```python
from build123d import *

# Parameters (mm, degrees)
SKETCH2_W           = 74.46
SKETCH2_H           = 52.500000064
SKETCH2_R           = 1
BOSS_EXTRUDE1_DEPTH = 2


with BuildPart() as part:
    # Sketch2 → Boss-Extrude1 (new body)
    with BuildSketch(Plane.XY):
        with Locations((51.585490461, 10.250000032)):
            Rectangle(SKETCH2_W, SKETCH2_H)
        with Locations((66.855490461, 35.000000064)):
            Circle(SKETCH2_R, mode=Mode.SUBTRACT)
        with Locations((15.855490461, 5.000000064)):
            Circle(SKETCH2_R, mode=Mode.SUBTRACT)
        with Locations((85.815490461, 35.000000064)):
            Circle(SKETCH2_R, mode=Mode.SUBTRACT)
        with Locations((85.815490461, -5.000000191)):
            Circle(SKETCH2_R, mode=Mode.SUBTRACT)
        with BuildLine():
            ThreePointArc((71.255490461, -4.000000191), (70.255490461, -5.000000191), (71.255490461, -6.000000191))
            ThreePointArc((71.255490461, -6.000000191), (72.255490461, -5.000000191), (71.255490461, -4.000000191))
        make_face(mode=Mode.SUBTRACT)
        with BuildLine():
            ThreePointArc((18.355490461, -13.5), (19.355490461, -14.5), (20.355490461, -13.5))
            ThreePointArc((20.355490461, -13.5), (19.355490461, -12.5), (18.355490461, -13.5))
        make_face(mode=Mode.SUBTRACT)
        with BuildLine():
            ThreePointArc((18.355490461, -8.5), (19.355490461, -9.5), (20.355490461, -8.5))
            ThreePointArc((20.355490461, -8.5), (19.355490461, -7.5), (18.355490461, -8.5))
        make_face(mode=Mode.SUBTRACT)
        with BuildLine():
            ThreePointArc((17.855490461, 0.500000064), (16.855490461, -0.499999936), (17.855490461, -1.499999936))
            ThreePointArc((17.855490461, -1.499999936), (18.855490461, -0.499999936), (17.855490461, 0.500000064))
        make_face(mode=Mode.SUBTRACT)
        with BuildLine():
            ThreePointArc((24.855490461, 0.500000064), (23.855490461, -0.499999936), (24.855490461, -1.499999936))
            ThreePointArc((24.855490461, -1.499999936), (25.855490461, -0.499999936), (24.855490461, 0.500000064))
        make_face(mode=Mode.SUBTRACT)
        with BuildLine():
            ThreePointArc((60.855490461, -13.5), (61.855490461, -14.5), (62.855490461, -13.5))
            ThreePointArc((62.855490461, -13.5), (61.855490461, -12.5), (60.855490461, -13.5))
        make_face(mode=Mode.SUBTRACT)
        with BuildLine():
            ThreePointArc((62.855490461, -8.5), (61.855490461, -7.5), (60.855490461, -8.5))
            ThreePointArc((60.855490461, -8.5), (61.855490461, -9.5), (62.855490461, -8.5))
        make_face(mode=Mode.SUBTRACT)
        with BuildLine():
            ThreePointArc((71.255490461, 34.000000064), (72.255490461, 35.000000064), (71.255490461, 36.000000064))
            ThreePointArc((71.255490461, 36.000000064), (70.255490461, 35.000000064), (71.255490461, 34.000000064))
        make_face(mode=Mode.SUBTRACT)
    extrude(amount=BOSS_EXTRUDE1_DEPTH)


solid = part.part
```
Check sheet for the modelled part. Datum: model origin and axes. Units: mm. Give positions to 0.01 mm unless a question says otherwise; leave off trailing zeros. Loops run counter-clockwise (first coordinate to the right, second up) from the corner with the lowest first, then second, coordinate; pieces in that order, holes last. Notation, with made-up numbers: M 19.25,1 L 34.25,1 A25 ccw 34.25,23 Z; hole C 3.5,74.5 d2. An arc over 180 degrees is marked long. Answer in a Markdown table with one row per item.
1) Mould release check, pull along Y, two halves, no side actions. Record for faces 1 (the face through (51, 36.5, 1)), 2 (the face through (88.815, 10, 1)), 3 (the face through (72.247, -4.87, 0.986)), 4 (the face through (18.62, -7.82, 0.99)): released by +Y, released by -Y, zero draft, split by the parting line, or undercut.
Solutions:
| item | result |
|---|---|
| face 1 | released by +Y |
| face 2 | zero draft |
| face 3 | undercut |
| face 4 | undercut |
2) Cross-section at A-A (y = 35). Enter the section's corners in (x, z).
Solutions:
| item | result |
|---|---|
| outline | M 14.36,0 L 65.86,0 L 65.86,2 L 14.36,2 Z; M 67.86,0 L 70.26,0 L 70.26,2 L 67.86,2 Z; M 72.26,0 L 84.82,0 L 84.82,2 L 72.26,2 Z; M 86.82,0 L 88.82,0 L 88.82,2 L 86.82,2 Z |
3) Cross-section at B-B (y = -0.5). Enter the section's corners in (x, z), plus the area to 3 significant figures.
Solutions:
| item | result |
|---|---|
| outline | M 14.36,0 L 16.86,0 L 16.86,2 L 14.36,2 Z; M 18.86,0 L 23.86,0 L 23.86,2 L 18.86,2 Z; M 25.86,0 L 88.82,0 L 88.82,2 L 25.86,2 Z |
| area | 141 mm^2 |
4) Thickness scan on line 1 (X direction, y = -0.5, z = 0.7); line 2 (Y direction, x = 25.5, z = 1.8). Record the ranges inside material, lowest first.
Solutions:
| item | result |
|---|---|
| line 1 | x = 14.36 to 16.86, 18.86 to 23.86, 25.86 to 88.82 |
| line 2 | y = -16 to -1.26, 0.26 to 36.5 |
5) Cross-section at C-C (y = 5). Enter the section's corners in (x, z), plus the area to 3 significant figures.
Solutions:
| item | result |
|---|---|
| outline | M 14.36,0 L 14.86,0 L 14.86,2 L 14.36,2 Z; M 16.86,0 L 88.82,0 L 88.82,2 L 16.86,2 Z |
| area | 145 mm^2 |
